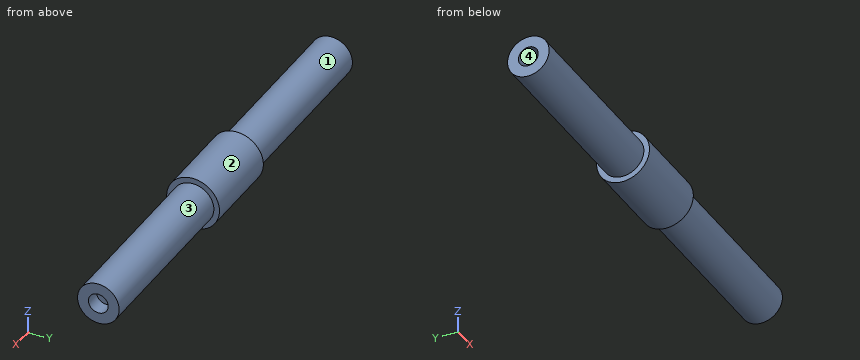
```python
from build123d import *

# Parameters (mm, degrees)
CROQUIS2_R            = 2.38125
CORTAR_EXTRUIR1_DEPTH = 10


with BuildPart() as part:
    # Croquis1 → Revolución1 (revolve)
    with BuildSketch(Plane(origin=(0, 0, 0), x_dir=(1, 0, 0), z_dir=(0, 1, 0))):
        Polygon((9.995, 6.35), (-10, 6.35), (-10, 5), (-53.175, 5), (-53.175, 0), (53.175, 0), (53.175, 5), (9.995, 5), align=None)
    revolve(axis=Axis((53.175, 0, 0), (-1, 0, 0)))

    # Croquis2 → Cortar-Extruir1 (cut)
    with BuildSketch(Plane.ZY.offset(53.175)):
        Circle(CROQUIS2_R)
    cortar_extruir1 = extrude(amount=-CORTAR_EXTRUIR1_DEPTH, mode=Mode.SUBTRACT)

    # Simetría1: Cortar-Extruir1 across plane
    add(cortar_extruir1.mirror(Plane.ZY.offset(-3.175)), mode=Mode.SUBTRACT)


solid = part.part
```
Could you check a few things on this model? Use its own coordinates, in mm. Face numbers are marked on the shaded views. A direction names the side the tool comes from. Round coordinates to 2 decimals unless told otherwise and drop trailing zeros. Order: outer loops, then holes, each group sorted by start corner. A loop starts at its lowest first (then second) coordinate and runs counter-clockwise, first axis right, second up. Notation, with made-up numbers: (-21.75, 42) -> (7.25, 42) arc R15 cw to (7.25, 67) -> close; hole circle Ø5 at (76.5, -3.5). An arc over 180 degrees is marked (long way). One line per question, with ' | ' between items.
Q1. If we section it at D-D on x = -2: Write out the boundary of the cut face in (y, z).
Computed values:
outline: circle Ø12.7 at (0, 0)
Q2. I'm going to push flat-ended pins straight in: pin 1 (4 mm diameter, centred on x = 33, y = 0.5, fed in from +Z); pin 2 (4 mm diameter, centred on y = 0, z = 0, fed in from -X) (3 decimals); pin 3 (1.4 mm diameter, centred on y = 0, z = 1, fed in from +X) (3 decimals). Where does each tip first touch, or does it pass through?
Computed values:
pin 1: z = 5 | pin 2: x = -43.175 | pin 3: x = 49.525
Q3. If we section it at A-A on y = 0: Write out the boundary of the cut face in (x, z) (3 decimals).
Computed values:
outline: (-53.175, -5) -> (-10, -5) -> (-10, -6.35) -> (9.995, -6.35) -> (9.995, -5) -> (53.175, -5) -> (53.175, -2.381) -> (49.525, -2.381) -> (49.525, 2.381) -> (53.175, 2.381) -> (53.175, 5) -> (9.995, 5) -> (9.995, 6.35) -> (-10, 6.35) -> (-10, 5) -> (-53.175, 5) -> (-53.175, 2.381) -> (-43.175, 2.381) -> (-43.175, -2.381) -> (-53.175, -2.381) -> close
Q4. If we section it at C-C on x = 31: Write out the boundary of the cut face in (y, z).
Computed values:
outline: circle Ø10 at (0, 0)
Q5. Which directions (+Z, -Z, +X, -X, +Y, -Y) give clear straight access to the entire face, cutting with the end or side of a thin tool? Please do the marked faces 1 and 2.
Computed values:
face 1: -X | face 2: +X, -X
Q6. If I drill on line 1 (Z direction, x = 51.15, y = 0); line 2 (X direction, y = 4.25, z = -4.5) (3 decimals), over which ranges is the centre line in solid material (lowest first)? Write a range as from..to.
Computed values:
line 1: -5..-2.38, 2.38..5 | line 2: -10..9.995
Q7. We'd pull the mould along Y, two halves only. Please class the marked faces 3 and 4: released by +Y, released by -Y, zero draft, split by the parting line, or undercut.
Computed values:
face 3: split by the parting line | face 4: undercut
